from build123d import *

# Parameters (mm, degrees)
SKETCH1_R             = 1.6
BOSS_EXTRUDE1_DEPTH   = 2
BOSS_EXTRUDE1_2_DEPTH = 2
SKETCH1_5_R           = 12.5
SKETCH1_5_R_2         = 9.5
BOSS_EXTRUDE2_DEPTH   = 8
SKETCH1_6_R           = 9.5
SKETCH1_6_R_2         = 4
BOSS_EXTRUDE3_DEPTH   = 2


with BuildPart() as part:
    # Sketch1 → Boss-Extrude1 (new body)
    with BuildSketch(Plane(origin=(0, 0, 0), x_dir=(0, 0, -1), z_dir=(1, 0, 0))):
        with BuildLine():
            Line((-5.859375, 11.041635957), (-18.34375, 4.416654383))
            ThreePointArc((-18.34375, 4.416654383), (-21, 0), (-18.34375, -4.416654383))
            Line((-18.34375, -4.416654383), (-5.859375, -11.041635957))
            ThreePointArc((-5.859375, -11.041635957), (-12.5, 0), (-5.859375, 11.041635957))
        make_face()
        with Locations((-16, 0)):
            Circle(SKETCH1_R, mode=Mode.SUBTRACT)
    extrude(amount=BOSS_EXTRUDE1_DEPTH)



with BuildPart() as body_2:
    # Sketch1 → Boss-Extrude1 2 (new body)
    with BuildSketch(Plane(origin=(0, 0, 0), x_dir=(0, 0, -1), z_dir=(1, 0, 0))):
        with BuildLine():
            Line((18.34375, 4.416654383), (5.859375, 11.041635957))
            ThreePointArc((5.859375, 11.041635957), (10.711960313, 6.44235254), (12.5, 0))
            ThreePointArc((12.5, 0), (10.711960313, -6.44235254), (5.859375, -11.041635957))
            Line((5.859375, -11.041635957), (18.34375, -4.416654383))
            ThreePointArc((18.34375, -4.416654383), (21, 0), (18.34375, 4.416654383))
        make_face()
        with Locations((16, 0)):
            Circle(SKETCH1_R, mode=Mode.SUBTRACT)
    extrude(amount=BOSS_EXTRUDE1_2_DEPTH)


with BuildPart() as part_1:
    add(part.part)

    add(body_2.part)  # Boss-Extrude2 merges body 2
    # Sketch1<5> → Boss-Extrude2 (add)
    with BuildSketch(Plane(origin=(0, 0, 0), x_dir=(0, 0, -1), z_dir=(1, 0, 0))):
        Circle(SKETCH1_5_R)
        Circle(SKETCH1_5_R_2, mode=Mode.SUBTRACT)
    extrude(amount=BOSS_EXTRUDE2_DEPTH)

    # Sketch1<6> → Boss-Extrude3 (add)
    with BuildSketch(Plane(origin=(0, 0, 0), x_dir=(0, 0, -1), z_dir=(1, 0, 0))):
        Circle(SKETCH1_6_R)
        Circle(SKETCH1_6_R_2, mode=Mode.SUBTRACT)
    extrude(amount=BOSS_EXTRUDE3_DEPTH)


solid = part_1.part
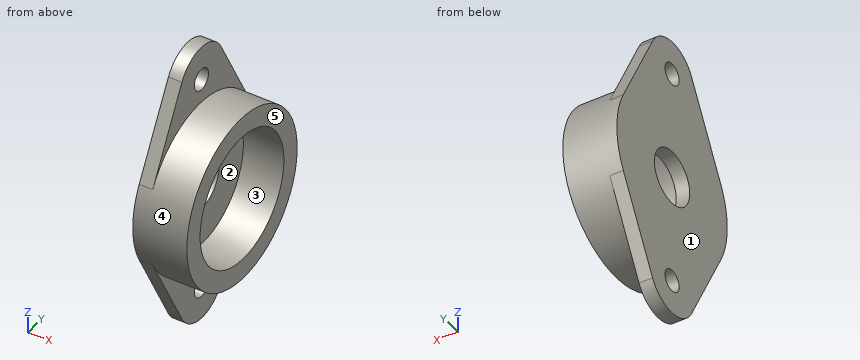
Check sheet for the modelled part. Datum: model origin and axes. Units: mm. Face numbers are marked on the shaded views. A direction names the side the tool comes from. Round coordinates to 2 decimals unless told otherwise and drop trailing zeros. Loops run counter-clockwise (first coordinate to the right, second up) from the corner with the lowest first, then second, coordinate; pieces in that order, holes last. Notation, with made-up numbers: (26.5, 47.5) -> (59.5, 47.5) arc R21 ccw to (59.5, 51.5) -> close; hole circle Ø1 at (-33.75, -5.5). An arc over 180 degrees is marked (long way). Put each result on its own line as item: value. Start each with the question number.
1. Section check C-C (x = 0.5). Enter the section's corners in (y, z).
2. Section check B-B (y = 0). Enter the section's corners in (x, z), plus the area to 3 significant figures.
3. Gauge pin test, flat ends, axial feed: pin 1 (4.5 mm diameter, centred on y = -1, z = -16, fed in from +X); pin 2 (4 mm diameter, centred on x = 1.5, z = -11, fed in from +Y) (3 decimals); pin 3 (1.5 mm diameter, centred on x = 4, y = 0.5, fed in from -Z). Record the tip position at first contact, or that the pin passes through.
4. Access from +Z, -Z, +X, -X, +Y, -Y to the whole of each face (thin tool, end or side, straight path). Record for the marked faces 1 and 2.
5. Section check A-A (z = 0). Enter the section's corners in (x, y).
6. Scan lines: probe 1 along Y at (x, z) = (0.5, 0); probe 2 along X at (y, z) = (-1.5, -18); probe 3 along Z at (x, y) = (6.75, -1). Record each from-to range of solid material in increasing order.
7. Draft check along Z on the marked faces 3, 4 and 5. Enter one of: +Z half, -Z half, draft (parallel to the pull), parting line (faces both ways), or undercut.
Findings:
1. outline: (-11.04, -5.86) -> (-4.42, -18.34) arc R5 ccw to (4.42, -18.34) -> (11.04, -5.86) arc R12.5 ccw to (11.04, 5.86) -> (4.42, 18.34) arc R5 ccw to (-4.42, 18.34) -> (-11.04, 5.86) arc R12.5 ccw to start; hole circle Ø8 at (0, 0); hole circle Ø3.2 at (0, -16); hole circle Ø3.2 at (0, 16)
2. outline: (0, -21) -> (2, -21) -> (2, -17.6) -> (0, -17.6) -> close; (0, -14.4) -> (2, -14.4) -> (2, -12.5) -> (8, -12.5) -> (8, -9.5) -> (2, -9.5) -> (2, -4) -> (0, -4) -> close; (0, 4) -> (2, 4) -> (2, 9.5) -> (8, 9.5) -> (8, 12.5) -> (2, 12.5) -> (2, 14.4) -> (0, 14.4) -> close; (0, 17.6) -> (2, 17.6) -> (2, 21) -> (0, 21) -> close
2. area: 91.2 mm^2
3. pin 1: stops at x = 2
3. pin 2: stops at y = 9.375
3. pin 3: stops at z = -12.5
4. face 1: +Z, -Z, -X, +Y, -Y
4. face 2: +X
5. outline: (0, -12.5) -> (8, -12.5) -> (8, -9.5) -> (2, -9.5) -> (2, -4) -> (0, -4) -> close; (0, 4) -> (2, 4) -> (2, 9.5) -> (8, 9.5) -> (8, 12.5) -> (0, 12.5) -> close
6. probe 1: y = -12.5 to -4, 4 to 12.5
6. probe 2: x = 0 to 2
6. probe 3: z = -12.46 to -9.45, 9.45 to 12.46
7. face 3: undercut
7. face 4: parting line
7. face 5: draft
